```python
from build123d import *

# Parameters (mm, degrees)
BOSS_EXTRUDE1_DEPTH = 9
SKETCH2_W           = 8
SKETCH2_H           = 9
BOSS_EXTRUDE2_DEPTH = 3
SKETCH3_W           = 3
SKETCH3_H           = 11
BOSS_EXTRUDE3_DEPTH = 2
SKETCH4_W           = 3
SKETCH4_H           = 11
BOSS_EXTRUDE4_DEPTH = 2
SKETCH6_W           = 34
SKETCH6_H           = 10
CUT_EXTRUDE2_DEPTH  = 3


with BuildPart() as part:
    # Sketch1 → Boss-Extrude1 (new body)
    with BuildSketch(Plane.XY):
        with BuildLine():
            Line((-10.712142643, -2.5), (-17, -2.5))
            Line((-17, -2.5), (-17, -24.5))
            Line((-17, -24.5), (17, -24.5))
            Line((17, -24.5), (17, -2.5))
            Line((17, -2.5), (10.712142643, -2.5))
            ThreePointArc((10.712142643, -2.5), (0, -11), (-10.712142643, -2.5))
        make_face()
    extrude(amount=BOSS_EXTRUDE1_DEPTH)

    # Sketch2 → Boss-Extrude2 (add)
    with BuildSketch(Plane.XZ.offset(24.5)):
        with Locations((0, 4.5)):
            Rectangle(SKETCH2_W, SKETCH2_H)
    extrude(amount=BOSS_EXTRUDE2_DEPTH)

    # Sketch3 → Boss-Extrude3 (add)
    with BuildSketch(Plane.ZY.offset(17)):
        with Locations((4.5, -19)):
            Rectangle(SKETCH3_W, SKETCH3_H)
    extrude(amount=BOSS_EXTRUDE3_DEPTH)

    # Sketch4 → Boss-Extrude4 (add)
    with BuildSketch(Plane(origin=(17, 0, 0), x_dir=(0, 0, -1), z_dir=(1, 0, 0))):
        with Locations((-4.5, -19)):
            Rectangle(SKETCH4_W, SKETCH4_H)
    extrude(amount=BOSS_EXTRUDE4_DEPTH)

    # Sketch6 → Cut-Extrude2 (cut)
    with BuildSketch(Plane.XY.offset(9)):
        with Locations((0, -22.5)):
            Rectangle(SKETCH6_W, SKETCH6_H)
    extrude(amount=-CUT_EXTRUDE2_DEPTH, mode=Mode.SUBTRACT)


solid = part.part
```
Could you check a few things on this model? Use its own coordinates, in mm. A direction names the side the tool comes from. Round coordinates to 2 decimals unless told otherwise and drop trailing zeros. Loops run counter-clockwise (first coordinate to the right, second up) from the corner with the lowest first, then second, coordinate; pieces in that order, holes last. Notation, with made-up numbers: (8, -16.75) - (19, -16.75) arc R20 ccw to (19, 13.25) - close; hole circle Ø6 at (67, 17.25). An arc over 180 degrees is marked (long way). Use CSV: the item, a comma, the result in double quotes.
Item 1: I need wall thicknesses on L1, parallel to Y at x = 13.5, z = 2.5; L2, parallel to Z at x = -15, y = -23.5; L3, parallel to X at y = -18, z = 1.75. Which ranges of each line are inside material? Lowest first, please. Write a range as [from, to].
Here are the results:
L1,"y = [-24.5, -2.5]"
L2,"z = [0, 6]"
L3,"x = [-17, 17]"
Item 2: If we section it at A-A on y = -6.75: List the corners of the cut face in (x, z) for me.
Here are the results:
outline,"(-17, 0) - (-8.69, 0) - (-8.69, 9) - (-17, 9) - close; (8.69, 0) - (17, 0) - (17, 9) - (8.69, 9) - close"
Item 3: Will these pins go through, and if not, where does the flat tip stop? pin 1 (4 mm diameter, centred on x = -7.5, z = 5.5, fed in from -Y); pin 2 (1.5 mm diameter, centred on y = -6, z = 8, fed in from +X); pin 3 (1 mm diameter, centred on x = 18, y = -20.5, fed in from -Z).
Here are the results:
pin 1,"stops at y = -24.5"
pin 2,"stops at x = 17"
pin 3,"stops at z = 3"
Item 4: If we section it at B-B on z = 5.5: List the corners of the cut face in (x, y) for me, then the cut area to 3 significant figures.
Here are the results:
outline,"(-19, -24.5) - (-4, -24.5) - (-4, -27.5) - (4, -27.5) - (4, -24.5) - (19, -24.5) - (19, -13.5) - (17, -13.5) - (17, -2.5) - (10.71, -2.5) arc R11 cw to (-10.71, -2.5) - (-17, -2.5) - (-17, -13.5) - (-19, -13.5) - close"
area,"680 mm²"
Item 5: If we section it at D-D on y = -23.25: List the corners of the cut face in (x, z) for me.
Here are the results:
outline,"(-19, 3) - (-17, 3) - (-17, 0) - (17, 0) - (17, 3) - (19, 3) - (19, 6) - (-19, 6) - close"
Item 6: For faces 1 (the flat face through (18, -19, 3)), 2 (the flat face through (0, -17.5, 8)), 3 (the flat face through (11, -24.5, 3)), which set-ups out of +Z, -Z, +X, -X, +Y, -Y let a thin tool reach every point of the face, with its end or its side?
Here are the results:
face 1,"-Z, +X, +Y, -Y"
face 2,"+Z, +X, -X, -Y"
face 3,"+Z, -Z, +X, -Y"
Item 7: If we section it at C-C on x = -12: List the corners of the cut face in (y, z) for me, then the cut area to 3 significant figures.
Here are the results:
outline,"(-24.5, 0) - (-2.5, 0) - (-2.5, 9) - (-17.5, 9) - (-17.5, 6) - (-24.5, 6) - close"
area,"177 mm²"
